Geometry: see drawing. Coordinates: mm, zero at the bounding-box minimum. A direction names the side the tool comes from. Round coordinates to 2 decimals unless told otherwise and drop trailing zeros. Order: outer loops, then holes, each group sorted by start corner. A loop starts at its lowest first (then second) coordinate and runs counter-clockwise, first axis right, second up. Notation, with made-up numbers: (5, -30) - (18, -30) arc R5 ccw to (18, -21) - close; hole circle Ø3 at (35, -34.75). An arc over 180 degrees is marked (long way). Put each result on its own line as item: value. Start each with the question number.
1) Contact query for flat-ended pins moving along their axis: P1, Ø3, axis at x = 3.5, z = 0.5, coming from the +Y side; P2, Ø2, axis at x = 2.5, y = 1.5, coming from the -Z side; P3, Ø1, axis at x = 11, y = 3, coming from the -Z side; P4, Ø3, axis at x = 7, y = 0.5, coming from the +Z side (1 decimal). Output: stop coordinate, or through.
2) Line query: probe 1 along Z at (x, y) = (9.25, 3.25); probe 2 along Y at (x, z) = (7, 2.55); probe 3 along X at (y, z) = (2.3, 3.85). Output: solid intervals per line, ascending. Write a range as [from, to].
3) Section B-B on x = 1.5. Output: boundary loops of the cut face in (y, z).
4) Access query for the marked faces 1 and 2. Directions: +Z, -Z, +X, -X, +Y, -Y. A direction counts if a zero-diameter tool reaches every point of the face in a straight line with its end or side. Return the directions, or none.
5) Section A-A on x = 6. Output: boundary loops of the cut face in (y, z).
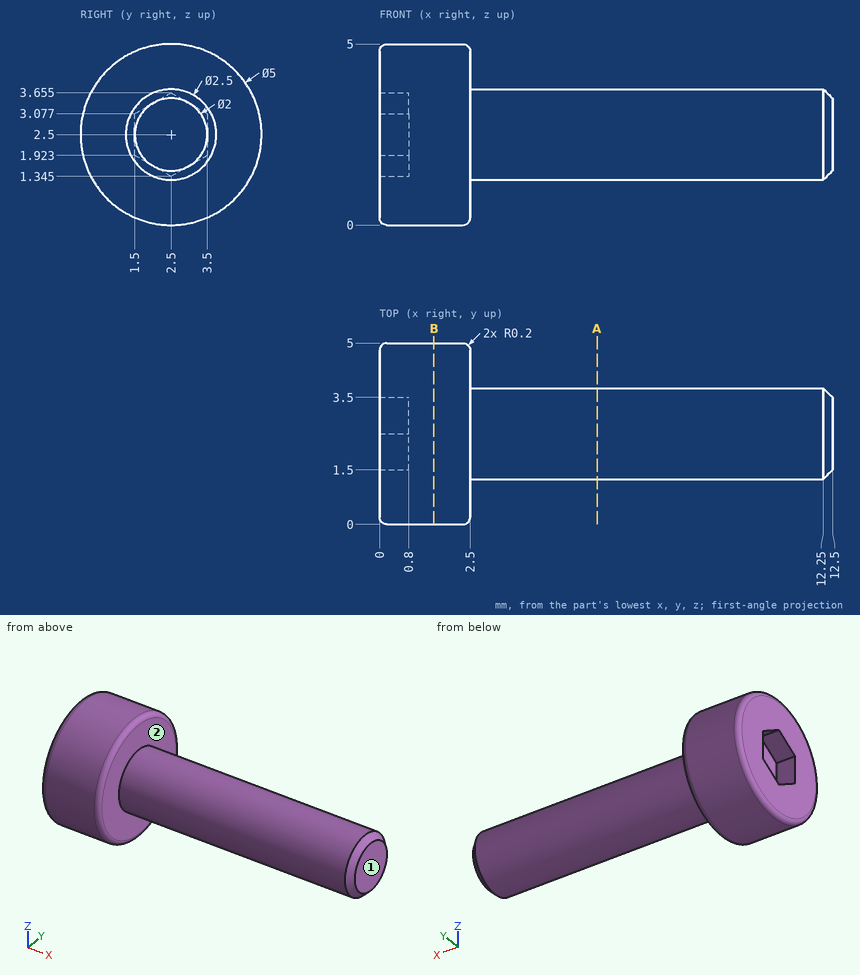
Answer sheet:
1. P1: y = 4.77
1. P2: z = 0
1. P3: z = 1.25
1. P4: z = 3.6
2. probe 1: [1.5, 3.5]
2. probe 2: [1.25, 3.75]
2. probe 3: [0, 2.5]
3. outline: circle Ø5 at (2.5, 2.5)
4. face 1: +Z, -Z, +X, +Y, -Y
4. face 2: +X
5. outline: circle Ø2.5 at (2.5, 2.5)
